Can you work these out from the drawing? Everything is in mm from the part's minimum corner. Give positions to 0.01 mm unless a question says otherwise; leave off trailing zeros. Order: outer loops, then holes, each group sorted by start corner. A loop starts at its lowest first (then second) coordinate and runs counter-clockwise, first axis right, second up. Notation, with made-up numbers: (79, 6.25) -> (121, 6.25) arc R27 ccw to (121, 27.25) -> close; hole circle Ø7 at (51.5, 19.25). An arc over 180 degrees is marked (long way). One line per item, written item: value.
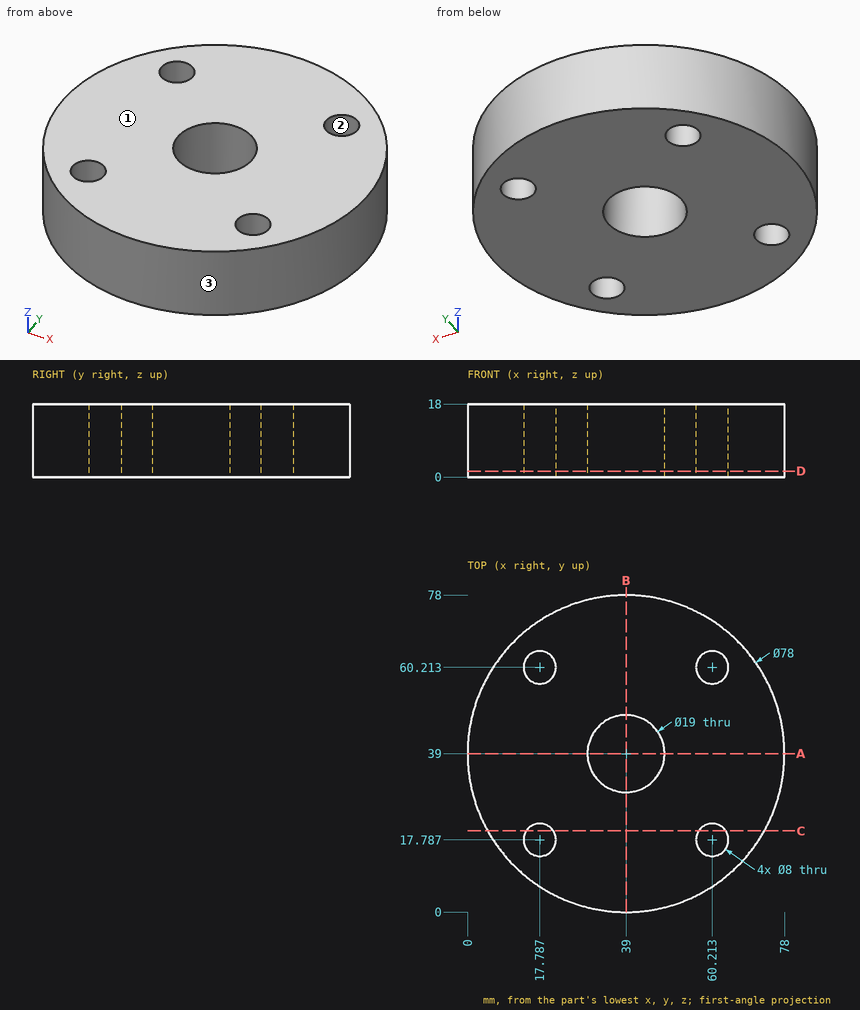
1) Suppose I cut it at C-C, the plane y = 20. Write out the boundary of the cut face in (x, z) (1 decimal).
Answer below:
outline: (4.9, 0) -> (14.5, 0) -> (14.5, 18) -> (4.9, 18) -> close; (21.1, 0) -> (56.9, 0) -> (56.9, 18) -> (21.1, 18) -> close; (63.5, 0) -> (73.1, 0) -> (73.1, 18) -> (63.5, 18) -> close
2) For P1, Ø2, axis at x = 42.5, z = 6, coming from the -Y side; P2, Ø1.5, axis at x = 10.5, z = 10.5, coming from the -Y side; P3, Ø1, axis at x = 42, z = 2.5, coming from the +Y side; P4, Ø8, axis at x = 27.5, y = 57, coming from the -Z side, each with a flat end and sliding along its axis, tell me the tip position at first contact or that it passes through.
Answer below:
P1: stops at y = 0.08
P2: stops at y = 11.6
P3: stops at y = 77.92
P4: stops at z = 0
3) Suppose I cut it at A-A, the plane y = 39. Write out the boundary of the cut face in (x, z), then the cut area to 3 significant figures.
Answer below:
outline: (0, 0) -> (29.5, 0) -> (29.5, 18) -> (0, 18) -> close; (48.5, 0) -> (78, 0) -> (78, 18) -> (48.5, 18) -> close
area: 1,060 mm2
4) If I drill on line 1 along Y through (x, z) = (39, 7.5); line 2 along Y through (x, z) = (61.5, 2.5) (1 decimal); line 3 along X through (y, z) = (57, 1) (1 decimal), over which ranges is the centre line in solid material (lowest first)?
Answer below:
line 1: y = 0 to 29.5, 48.5 to 78
line 2: y = 7.1 to 14, 21.6 to 56.4, 64 to 70.9
line 3: x = 4.4 to 15.4, 20.2 to 57.8, 62.6 to 73.6
5) We'd pull the mould along Y, two halves only. Please class the marked faces 1, 2 and 3: +Y half, -Y half, draft (parallel to the pull), parting line (faces both ways), or undercut.
Answer below:
face 1: draft
face 2: undercut
face 3: parting line
6) Suppose I cut it at D-D, the plane z = 1.5. Write out the boundary of the cut face in (x, y), then the cut area to 3 significant figures.
Answer below:
outline: circle Ø78 at (39, 39); hole circle Ø8 at (17.79, 17.79); hole circle Ø8 at (17.79, 60.21); hole circle Ø19 at (39, 39); hole circle Ø8 at (60.21, 17.79); hole circle Ø8 at (60.21, 60.21)
area: 4,290 mm2
